Autodesk Inventor part; units mm, degrees
ref_plane "YZ Plane" through (0, 0, 0) normal (1, 0, 0) x (0, 1, 0)
ref_plane "XZ Plane" through (0, 0, 0) normal (0, 1, 0) x (-1, 0, 0)
ref_plane "XY Plane" through (0, 0, 0) normal (0, 0, 1) x (1, 0, 0)
sketch "Sketch1" plane through (0, 0, 0) normal (0, 0, 1) x (1, 0, 0)
  circle A0 centre (0, 0) radius 35
  dimension "d0" = 70
extrude "Extrusion1" add sketch "Sketch1" along normal blind 3
sketch "Sketch2" plane through (0, 0, 3) normal (0, 0, 1) x (1, 0, 0)
  circle A0 centre (0, 0) radius 32 construction
  point P0 (32, 0)
  dimension "d3" = 64
hole "Hole1" at (32, 0, 3) direction (0, 0, -1) diameter 3.4 depth 10 tip angle 118
pattern_circular "Circular Pattern1" count 4 over 360 about axis through (0, 0, 0) along (0, 0, 1) of "Hole1"
hole "Hole2" at (0, 0, 0) direction (0, 0, 1) diameter 6.2 end through all
properties part number "anode_holder" material "Copper"
Part model, mm, in its own coordinate system. Give positions to 0.01 mm unless a question says otherwise; leave off trailing zeros. Loops run counter-clockwise (first coordinate to the right, second up) from the corner with the lowest first, then second, coordinate; pieces in that order, holes last. Notation, with made-up numbers: M 69,-18 L 99,-18 A23 cw 99,-4 Z; hole C 65,-11.5 d6. An arc over 180 degrees is marked long. Return JSON: item names as keys, results as strings.
1) Flat gauge pin, fed straight in: pin 1 Ø4 at (x, y) = (-15, -14) entering from -Z. Where does the tip first touch, or does it go through?
Calculated:
{"pin 1": "stops at z = 0"}
2) Drill centre lines: line 1 (Y direction, x = 0, z = 0.9); line 2 (Y direction, x = -2, z = 1.55); line 3 (Y direction, x = 2.5, z = 0.75). Where is each one in solid material? Low to high.
Calculated:
{"line 1": "y = -35 to -33.7, -30.3 to -3.1, 3.1 to 30.3, 33.7 to 35", "line 2": "y = -34.94 to -2.37, 2.37 to 34.94", "line 3": "y = -34.91 to -1.83, 1.83 to 34.91"}
3) Saw through at D-D, the plane x = 32. List the corners of the cut face in (y, z), then the cut area to 3 significant figures.
Calculated:
{"outline": "M -14.18,0 L -1.7,0 L -1.7,3 L -14.18,3 Z; M 1.7,0 L 14.18,0 L 14.18,3 L 1.7,3 Z", "area": "74.9 mm2"}
4) Pull direction X, two halves, no side cores. Call faces 1 (the face through (0, -7, 0)), 2 (the face through (33.66, 0.37, 1.48)), 3 (the face through (-28, 21, 1)): released by +X, released by -X, zero draft, split by the parting line, or undercut.
Calculated:
{"face 1": "zero draft", "face 2": "undercut", "face 3": "split by the parting line"}
5) Saw through at A-A, the plane x = 0. List the corners of the cut face in (y, z), then the cut area to 3 significant figures.
Calculated:
{"outline": "M -35,0 L -33.7,0 L -33.7,3 L -35,3 Z; M -30.3,0 L -3.1,0 L -3.1,3 L -30.3,3 Z; M 3.1,0 L 30.3,0 L 30.3,3 L 3.1,3 Z; M 33.7,0 L 35,0 L 35,3 L 33.7,3 Z", "area": "171 mm2"}
6) Saw through at C-C, the plane z = 0.95. List the corners of the cut face in (x, y).
Calculated:
{"outline": "C 0,0 d70; hole C -32,0 d3.4; hole C 0,0 d6.2; hole C 0,-32 d3.4; hole C 0,32 d3.4; hole C 32,0 d3.4"}
